Source: CAD feature listing. Evaluate the final solid. Frame: model axes, mm. Give positions to 0.01 mm unless a question says otherwise; leave off trailing zeros. Loops run counter-clockwise (first coordinate to the right, second up) from the corner with the lowest first, then second, coordinate; pieces in that order, holes last. Notation, with made-up numbers: M 84.25,89.5 L 138.25,89.5 A10 cw 138.25,95.5 Z; hole C -4.75,74 d7. An arc over 180 degrees is marked long. Put each result on its own line as item: value.
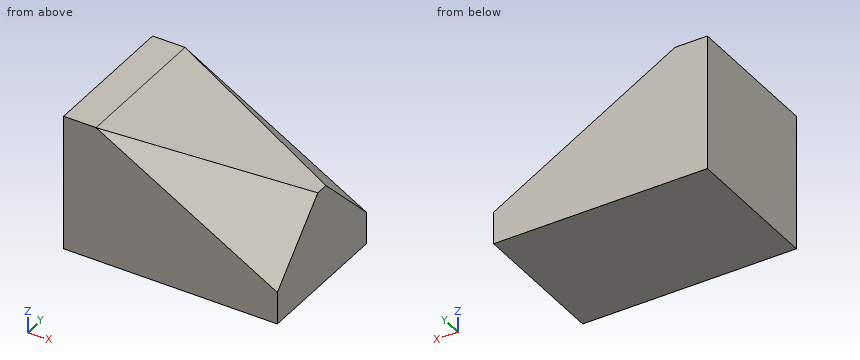
Autodesk Inventor part; units mm, degrees
ref_plane "工作平面1" through (10, 22, 0) normal (-0.3746, -0.6556, -0.6556) x (0.8682, 0, -0.4961)
ref_plane "YZ Plane" through (0, 0, 0) normal (1, 0, 0) x (0, 1, 0)
ref_plane "XZ Plane" through (0, 0, 0) normal (0, 1, 0) x (-1, 0, 0)
sketch "草圖1" plane through (0, 0, 0) normal (0, 1, 0) x (-1, 0, 0)
  line L0 (0, 0) -> (-66, 0)
  line L1 (-66, 0) -> (-66, -42)
  line L2 (-66, -42) -> (0, -42)
  line L3 (0, -42) -> (0, 0)
  dimension "d0" = 66
  dimension "d1" = 42
extrude "擠出1" add sketch "草圖1" along normal mid plane 44
sketch "草圖2" plane through (0, 22, 0) normal (0, 1, 0) x (1, 0, 0)
  line L0 (0, 0) -> (66, 0)
  line L1 (10, 0) -> (66, 12)
  line L2 (66, 0) -> (66, 42)
  dimension "d4" = 10
  dimension "d5" = 30
extrude "擠出2" cut sketch "草圖2" against normal blind 60
sketch "草圖3" plane through (66, -22, -42) normal (1, 0, 0) x (0, 0, -1)
  line L0 (-30, 24) -> (-10, 44)
  line L1 (0, 44) -> (-42, 44)
  line L2 (-30, 44) -> (-30, 0)
  point P0 (-42, 22)
  point P1 (-30, 2)
  dimension "d8" = 20
  dimension "d9" = 20
ref_plane "工作平面1" through (10, 22, 0) normal (-0.3746, -0.6556, -0.6556) x (0.8682, 0, -0.4961)
sketch "草圖4" plane through (10, 22, 0) normal (-0.3746, -0.6556, -0.6556) x (0.8682, 0, -0.4961)
  line L0 (-15.1543, -12.3218) -> (93.717, -12.3218)
  line L1 (93.717, -12.3218) -> (93.717, 28.8166)
  line L2 (93.717, 28.8166) -> (-15.1543, 28.8166)
  line L3 (-15.1543, 28.8166) -> (-15.1543, -12.3218)
  point P0 (-8.6824, 13.3595)
extrude "擠出3" cut sketch "草圖4" against normal blind 40
mirror "鏡射1" about plane through (0, 0, 0) normal (0, 1, 0) of "擠出3"
properties part number "60"
1. Material intervals for line 1 (Z direction, x = 21, y = 1.5); line 2 (Z direction, x = 57, y = -20); line 3 (Y direction, x = 58, z = -16.5), sorted ascending. Write a range as from..to.
Found:
line 1: -42..-2.36
line 2: -42..-24.86
line 3: -11.07..11.07
2. Section query B-B (z = -3). Output: boundary loops of the cut face in (x, y).
Found:
outline: M 0,-22 L 15.25,-22 L 24,-17 L 24,17 L 15.25,22 L 0,22 Z
3. Contact query for flat-ended pins moving along their axis: P1, Ø10, axis at y = -9, z = -17, coming from the -X side; P2, Ø3, axis at x = 34.5, z = -5, coming from the -Y side; P3, Ø5, axis at x = 31, y = -9, coming from the +Z side. Output: stop coordinate, or through.
Found:
P1: x = 0
P2: y = -14.73
P3: z = -3.96
4. Section query A-A (y = 8). Output: boundary loops of the cut face in (x, z), plus the area to 3 significant figures.
Found:
outline: M 0,-42 L 66,-42 L 66,-18 L 49.2,-8.4 L 10,0 L 0,0 Z
area: 2,390 mm^2
